The listing builds one solid part. Answer for the finished solid, in the listing's coordinates (mm). Give positions to 0.01 mm unless a question says otherwise; leave off trailing zeros. Loops run counter-clockwise (first coordinate to the right, second up) from the corner with the lowest first, then second, coordinate; pieces in that order, holes last. Notation, with made-up numbers: M -28.5,-34 L 22.5,-34 A23 ccw 22.5,-25 Z; hole C -4.5,34.25 d5. An arc over 180 degrees is marked long. Use one line per item in the form item = value. Start each with the question number.
1. The part is cut by section A-A (y = 10). Write down the section's boundary in (x, z).
2. Straight lines are drawn through the part: line 1 (Y direction, x = -37.7, z = 11); line 2 (Z direction, x = -37.7, y = 10); line 3 (Z direction, x = -38.2, y = 8). For each, find the intervals that lie inside material, in ascending order. Write a range as from..to.
3. The part is cut by section C-C (x = -37.75). Write down the section's boundary in (y, z).
4. The part is cut by section B-B (z = 11). Write down the section's boundary in (x, y), and give its area (3 significant figures).
5. This flat-tipped pin is pushed along its axis until it touches: pin 1 Ø4 at (y, z) = (10, 11) entering from -X. Where does it stop, or does it pass through?
6. The part is cut by section D-D (z = 7). Write down the section's boundary in (x, y), and give its area (3 significant figures).
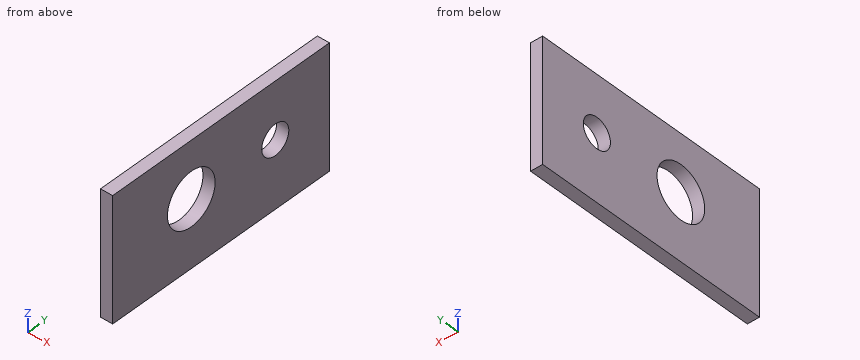
from build123d import *

# Parameters (mm, degrees)
SKETCH006_W    = 16
SKETCH006_H    = 5.3
SKETCH006_W_2  = 5.6
SKETCH006_H_2  = 4.4
CYLINDER_R     = 2.5
CYLINDER_DEPTH = 10
SKETCH_W       = 40
SKETCH_H       = 20.3
PAD005_DEPTH   = 2


with BuildPart() as power_socket_mockup:
    # Sketch006 → Revolution (revolve)
    with BuildSketch(Plane.XZ):
        with Locations((8, -2.65)):
            Rectangle(SKETCH006_W, SKETCH006_H)
        with Locations((-2.8, -2.2)):
            Rectangle(SKETCH006_W_2, SKETCH006_H_2)
    revolve(axis=Axis((0, 0, 0), (1, 0, 0)))


with BuildPart() as power_socket_mockup_1:
    # Body005 placement: moved
    add(power_socket_mockup.part.moved(Location((-36, -5.5, 11))))


with BuildPart() as wire_hole:
    # Cylinder → Cylinder (new body)
    with BuildSketch(Plane(origin=(-41, 10, 11), x_dir=(0, 0, -1), z_dir=(1, 0, 0))):
        Circle(CYLINDER_R)
    extrude(amount=CYLINDER_DEPTH)


with BuildPart() as power_holes_cut:
    # Sketch → Pad005 (new body)
    with BuildSketch(Plane.YZ.offset(28.5)):
        with Locations((0, 10.15)):
            Rectangle(SKETCH_W, SKETCH_H)
    extrude(amount=PAD005_DEPTH)


with BuildPart() as power_holes_cut_1:
    # Body003 placement: moved
    add(power_holes_cut.part.moved(Location((-67, 0, 0))))

    # Cut: cut wire_hole
    add(wire_hole.part, mode=Mode.SUBTRACT)

    # Cut002: cut power socket mockup
    add(power_socket_mockup_1.part, mode=Mode.SUBTRACT)


solid = power_holes_cut_1.part
Derived:
q1.outline = M -38.5,0 L -36.5,0 L -36.5,8.5 L -38.5,8.5 Z; M -38.5,13.5 L -36.5,13.5 L -36.5,20.3 L -38.5,20.3 Z
q2.line_1 = -20..-9.9, -1.1..7.5, 12.5..20
q2.line_2 = 0..8.5, 13.5..20.3
q2.line_3 = 0..9.5, 12.5..20.3
q3.outline = M -20,0 L 20,0 L 20,20.3 L -20,20.3 Z; hole C -5.5,11 d8.8; hole C 10,11 d5
q4.outline = M -38.5,-20 L -36.5,-20 L -36.5,-9.9 L -38.5,-9.9 Z; M -38.5,-1.1 L -36.5,-1.1 L -36.5,7.5 L -38.5,7.5 Z; M -38.5,12.5 L -36.5,12.5 L -36.5,20 L -38.5,20 Z
q4.area = 52.4 mm2
q5.pin_1 = through
q6.outline = M -38.5,-20 L -36.5,-20 L -36.5,-7.33 L -38.5,-7.33 Z; M -38.5,-3.67 L -36.5,-3.67 L -36.5,20 L -38.5,20 Z
q6.area = 72.7 mm2
